The model under review builds one solid part; all positions refer to its coordinate system, in mm. Give positions to 0.01 mm unless a question says otherwise; leave off trailing zeros. Loops run counter-clockwise (first coordinate to the right, second up) from the corner with the lowest first, then second, coordinate; pieces in that order, holes last. Notation, with made-up numbers: M 7,15 L 44,15 A29 ccw 44,38 Z; hole C 50.25,84.5 d7. An arc over 180 degrees is marked long. One line per item, written item: value. Start each with the question number.
Q1. We need section D-D on x = -23.5. Write out the cut boundary in (y, z).
Q2. We need section C-C on z = 110.5. Write out the cut boundary in (x, y).
Q3. We need section B-B on y = -2.5. Give the number of separate pieces and of enclosed holes in the cut face, plus the area to 3 significant figures.
Q4. To check wall thickness, follow line 1 along Z through (x, y) = (-8.5, -1.75); line 2 along Z through (x, y) = (11.5, -2.5); line 3 along Z through (x, y) = (-15.5, -7). State the ranges of each line that lie inside material, in increasing order. Write a range as from..to.
Q5. We need section A-A on x = 13.5. Write out the cut boundary in (y, z) (3 decimals), plus the area to 3 significant figures.
Q6. For pin 1 (2.5 mm diameter, centred on y = -7, z = -45.5, fed in from +X); pin 2 (0.9 mm diameter, centred on x = -5.5, y = -6.5, fed in from -Z); pin 3 (3 mm diameter, centred on x = -8, z = -47.5, fed in from +Y); pin 4 (16.5 mm diameter, centred on x = 13.5, z = -46, fed in from -Y), all flat-tipped, find the tip position at first contact; note any pin that passes through.
```python
from build123d import *

# Parameters (mm, degrees)
F0_W      = 35
F0_H      = 200
F1_DEPTH  = 8
F2_R      = 6.075
F3_DEPTH  = 45
F4_W      = 6
F4_H      = 2
F6_DEPTH  = 25
F7_R      = 0.3
F8_R      = 3.25
F9_DEPTH  = 25
F10_R     = 3.25
F11_DEPTH = 4
F12_R     = 3.25
F13_DEPTH = 3
F14_W     = 3
F14_H     = 15
F15_DEPTH = 3
F18_DEPTH = 8
F20_DEPTH = 65
F21_W     = 6
F21_H     = 2
F22_DEPTH = 25
F23_R     = 4


with BuildPart() as f1:
    # F0 (on Front) → F1 (new body)
    with BuildSketch(Plane.XZ):
        with Locations((4.1207429767, 45.2379755676)):
            Rectangle(F0_W, F0_H)
    extrude(amount=F1_DEPTH)

    # F2 (on face) → F3 (cut)
    with BuildSketch(Plane(origin=(-13.3792570233, 0, 0), x_dir=(0, -1, 0), z_dir=(-1, 0, 0))):
        with Locations((0, 137.2379755676)):
            Circle(F2_R)
    extrude(amount=-F3_DEPTH, mode=Mode.SUBTRACT)

    # F4 (on face) → F6 (cut)
    with BuildSketch(Plane(origin=(0, 0, 0), x_dir=(-1, 0, 0), z_dir=(0, 1, 0))):
        with Locations((-4.1207429767, 128.1629755676)):
            Rectangle(F4_W, F4_H)
    extrude(amount=-F6_DEPTH, mode=Mode.SUBTRACT)

    # F7
    f7_edges = [f1.edges().sort_by_distance(p)[0] for p in [
        (4.120743, -8, 129.162976),
        (4.120743, -8, 127.162976),
        (7.120743, -8, 128.162976),
        (1.120743, -8, 128.162976),
        (4.120743, 0, 129.162976),
        (7.120743, 0, 128.162976),
        (4.120743, 0, 127.162976),
        (1.120743, 0, 128.162976),
    ]]
    fillet(f7_edges, radius=F7_R)

    # F8 (on face) → F9 (cut)
    with BuildSketch(Plane.XZ.offset(8)):
        with Locations((-5.3792570233, -47.7620244324)):
            Circle(F8_R)
        with Locations((13.6207429767, -47.7620244324)):
            Circle(F8_R)
    extrude(amount=-F9_DEPTH, mode=Mode.SUBTRACT)

    # F10 (on face) → F11 (cut)
    with BuildSketch(Plane(origin=(0, 0, 0), x_dir=(-1, 0, 0), z_dir=(0, 1, 0))):
        Polygon((-10.593553136, -52.9423836544), (-7.6208253694, -47.7305807393), (-10.64801521, -42.5502215174), (-16.6479328173, -42.5816652105), (-19.6206605839, -47.7934681255), (-16.5934707433, -52.9738273475), align=None)
        with Locations((-13.6207429767, -47.7620244324)):
            Circle(F10_R, mode=Mode.SUBTRACT)
        Polygon((8.4202988823, -52.9342642192), (11.3790690026, -47.7145248219), (8.3380271436, -42.5422850352), (2.3382151643, -42.5897846457), (-0.620554956, -47.8095240429), (2.420486903, -52.9817638297), align=None)
        with Locations((5.3792570233, -47.7620244324)):
            Circle(F10_R, mode=Mode.SUBTRACT)
    extrude(amount=-F11_DEPTH, mode=Mode.SUBTRACT)

    # F12 (on face) → F13 (cut)
    with BuildSketch(Plane.XZ.offset(8)):
        Polygon((-13.3792570233, -40.5933335423), (-13.3792570233, -54.7620244324), (21.6207429767, -54.7620244324), (21.6207429767, -40.5933335423), (21.6207429767, -39.7620244324), (-13.3792570233, -39.7620244324), align=None)
        with Locations((-5.3792570233, -47.7620244324)):
            Circle(F12_R, mode=Mode.SUBTRACT)
        with Locations((13.6207429767, -47.7620244324)):
            Circle(F12_R, mode=Mode.SUBTRACT)
        Polygon((-13.3792570233, -40.5933335423), (-13.3792570233, -54.7620244324), (21.6207429767, -54.7620244324), (21.6207429767, -40.5933335423), (21.6207429767, -39.7620244324), (-13.3792570233, -39.7620244324), align=None)
    extrude(amount=-F13_DEPTH, mode=Mode.SUBTRACT)

    # F14 (on face) → F15 (join)
    with BuildSketch(Plane.XZ.offset(5)):
        with Locations((4.1207429767, -47.2620244324)):
            Rectangle(F14_W, F14_H)
    extrude(amount=F15_DEPTH)

    # F16 (on face) → F18 (join)
    with BuildSketch(Plane.XZ.offset(8)):
        with BuildLine():
            Line((-35.1568526326, 39.9309880875), (-34.2461589726, 39.1493094232))
            ThreePointArc((-34.2461589726, 39.1493094232), (-33.657494289, 39.8672680482), (-33.1251321385, 40.6279133253))
            Line((-33.1251321385, 40.6279133253), (-13.3792570233, 33.3985724449))
            Line((-13.3792570233, 33.3985724449), (-13.3792570233, 61.0773786902))
            Line((-13.3792570233, 61.0773786902), (-33.1251321385, 53.8480378099))
            ThreePointArc((-33.1251321385, 53.8480378099), (-42.6403240796, 59.4155770599), (-52.7588970229, 55.0394083513))
            Line((-52.7588970229, 55.0394083513), (-51.8482033629, 54.257729687))
            ThreePointArc((-51.8482033629, 54.257729687), (-36.2148256468, 55.5848865562), (-35.1568526326, 39.9309880875))
        make_face()
    extrude(amount=-F18_DEPTH)

    # F19 (on face) → F20 (cut)
    with BuildSketch(Plane.YZ.offset(21.6207429767)):
        with BuildLine():
            ThreePointArc((-8, 41.585023515), (-5.1010205144, 43.7777761493), (-4, 47.2418777645))
            ThreePointArc((-4, 47.2418777645), (-5.1010205144, 50.7059793796), (-8, 52.898732014))
            Line((-8, 52.898732014), (-8, 41.585023515))
        make_face()
    extrude(amount=-F20_DEPTH, mode=Mode.SUBTRACT)

    # F21 (on face) → F22 (cut)
    with BuildSketch(Plane.XZ.offset(8)):
        with Locations((4.1207429767, 39.585023515)):
            Rectangle(F21_W, F21_H)
        with Locations((4.1207429767, 54.898732014)):
            Rectangle(F21_W, F21_H)
    extrude(amount=-F22_DEPTH, mode=Mode.SUBTRACT)

    # F23
    f23_edges = [f1.edges().sort_by_distance(p)[0] for p in [
        (4.120743, 0, 40.585024),
        (4.120743, 0, 53.898732),
    ]]
    fillet(f23_edges, radius=F23_R)


solid = f1.part
```
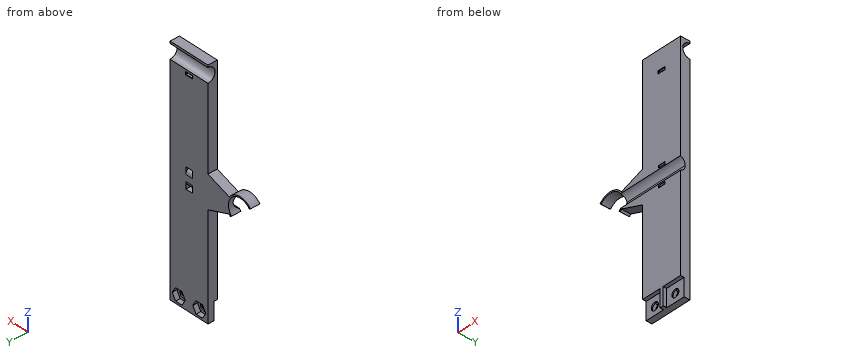
Solved:
1. outline: M -8,37.1 L 0,37.1 L 0,57.37 L -8,57.37 L -8,52.9 A6 cw -8,41.59 Z
2. outline: M -13.38,-8 L 21.62,-8 L 21.62,0 L -13.38,0 Z
3. separate pieces: 2
3. enclosed holes: 5
3. area: 6,820 mm2
4. line 1: -54.76..-52.79, -42.82..131.42, 143.06..145.24
4. line 2: -54.76..-52.95, -42.55..131.7, 142.77..145.24
4. line 3: 34.18..42.05, 52.44..60.3
5. outline: M -8,-39.762 L -5,-39.762 L -5,-44.514 L -4,-44.514 L -4,-42.565 L 0,-42.565 L 0,131.163 A6.075 cw 0,143.313 L 0,145.238 L -8,145.238 L -8,52.899 A6 cw -8,41.585 Z; M -5,-54.762 L 0,-54.762 L 0,-52.958 L -4,-52.958 L -4,-51.01 L -5,-51.01 Z
5. area: 1,420 mm2
6. pin 1: x = 5.62
6. pin 2: z = -39.76
6. pin 3: y = -4
6. pin 4: y = -8
